The model under review builds one solid part; all positions refer to its coordinate system, in mm. Face numbers are marked on the shaded views. A direction names the side the tool comes from. Coordinates: 2 decimals unless noted, no trailing zeros. Write each loop counter-clockwise with the first axis right and the second up, starting at its lowest first coordinate (ties: lowest second). Pieces come first, ordered by that corner, then holes.
```python
from build123d import *

# Parameters (mm, degrees)
EXTRUDE_1_DEPTH = 2
SKETCH_3_W      = 3.4
SKETCH_3_H      = 17
EXTRUDE_2_DEPTH = 15
SKETCH_6_W      = 5
SKETCH_6_H      = 9
EXTRUDE_4_DEPTH = 2


with BuildPart() as part:
    # 스케치1 → 보스-돌출1 (new body)
    with BuildSketch(Plane.XY):
        with BuildLine():
            Line((30.660415516, 8.5), (70.121524493, 22.5))
            Line((70.121524493, 22.5), (75.121524493, 22.5))
            Line((75.121524493, 22.5), (75.121524493, 13.5))
            Line((75.121524493, 13.5), (70.121524493, 13.5))
            Line((70.121524493, 13.5), (30.660415516, 0.952987126))
            ThreePointArc((30.660415516, 0.952987126), (29.963426304, 0), (30.660415516, -0.952987126))
            Line((30.660415516, -0.952987126), (70.121524493, -13.5))
            Line((70.121524493, -13.5), (75.121524493, -13.5))
            Line((75.121524493, -13.5), (75.121524493, -22.5))
            Line((75.121524493, -22.5), (70.121524493, -22.5))
            Line((70.121524493, -22.5), (30.660415516, -8.5))
            Line((30.660415516, -8.5), (-3.878475507, -8.5))
            Line((-3.878475507, -8.5), (-3.878475507, 8.5))
            Line((-3.878475507, 8.5), (30.660415516, 8.5))
        make_face()
    extrude(amount=EXTRUDE_1_DEPTH)

    # 스케치3 → 보스-돌출2 (add)
    with BuildSketch(Plane(origin=(0, 0, 0), x_dir=(-1, 0, 0), z_dir=(0, 0, -1))):
        with Locations((2.178475507, 0)):
            Rectangle(SKETCH_3_W, SKETCH_3_H)
    extrude(amount=EXTRUDE_2_DEPTH)

    # 스케치6 → 보스-돌출4 (add)
    with BuildSketch(Plane(origin=(0, 0, 0), x_dir=(-1, 0, 0), z_dir=(0, 0, -1))):
        with Locations((-72.621524493, -18)):
            Rectangle(SKETCH_6_W, SKETCH_6_H)
        with Locations((-72.621524493, 18)):
            Rectangle(SKETCH_6_W, SKETCH_6_H)
    extrude(amount=EXTRUDE_4_DEPTH)


solid = part.part
```
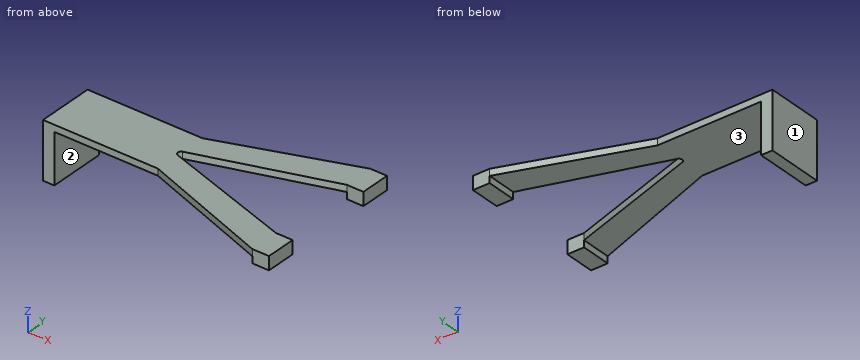
Item 1: Take a section at D-D, the plane x = 39.5. Write out the cut boundary in (y, z).
Solved:
outline: (-11.64, 0) - (-3.76, 0) - (-3.76, 2) - (-11.64, 2) - close; (3.76, 0) - (11.64, 0) - (11.64, 2) - (3.76, 2) - close
Item 2: Take a section at B-B, the plane x = 52. Write out the cut boundary in (y, z), plus the area to 3 significant figures.
Solved:
outline: (-16.07, 0) - (-7.74, 0) - (-7.74, 2) - (-16.07, 2) - close; (7.74, 0) - (16.07, 0) - (16.07, 2) - (7.74, 2) - close
area: 33.3 mm2
Item 3: To check wall thickness, follow line 1 along Z through (x, y) = (19.5, -1); line 2 along X through (y, z) = (1, -8.25). State the ranges of each line that lie inside material, in increasing order.
Solved:
line 1: z = 0 to 2
line 2: x = -3.88 to -0.48
Item 4: For pin 1 (13.5 mm diameter, centred on x = 37.5, y = -1.5, fed in from -Z); pin 2 (0.6 mm diameter, centred on y = -19.5, z = -1.5, fed in from -X); pin 3 (4.5 mm diameter, centred on y = -3, z = -5, fed in from +X), all flat-tipped, find the tip position at first contact; note any pin that passes through.
Solved:
pin 1: stops at z = 0
pin 2: stops at x = 70.12
pin 3: stops at x = -0.48
Item 5: Take a section at A-A, the plane z = -1.25. Write out the cut boundary in (x, y).
Solved:
outline: (-3.88, -8.5) - (-0.48, -8.5) - (-0.48, 8.5) - (-3.88, 8.5) - close; (70.12, -22.5) - (75.12, -22.5) - (75.12, -13.5) - (70.12, -13.5) - close; (70.12, 13.5) - (75.12, 13.5) - (75.12, 22.5) - (70.12, 22.5) - close
Item 6: Machinability: for the marked faces 1, 2 and 3, which of the approach directions +Z, -Z, +X, -X, +Y, -Y give a long, thin tool a straight path to every point of the face, cutting with its end or side? Answer none if there is none.
Solved:
face 1: +Z, -Z, -X, +Y, -Y
face 2: -Z, +X, +Y, -Y
face 3: -Z, +Y, -Y
Item 7: Take a section at C-C, the plane z = -6.25. Write out the cut boundary in (x, y), plus the area to 3 significant figures.
Solved:
outline: (-3.88, -8.5) - (-0.48, -8.5) - (-0.48, 8.5) - (-3.88, 8.5) - close
area: 57.8 mm2
